Source: CAD feature listing. Evaluate the final solid. Frame: model axes, mm. Face numbers are marked on the shaded views. A direction names the side the tool comes from. Coordinates: 2 decimals unless noted, no trailing zeros. Loops run counter-clockwise (first coordinate to the right, second up) from the corner with the lowest first, then second, coordinate; pieces in that order, holes last.
Item 1: Pin query (flat end, axial travel): pin 1 Ø0.8 at (x, z) = (2.5, 16.5) entering from +Y; pin 2 Ø0.8 at (x, z) = (-3, 22) entering from -Y; pin 3 Ø2 at (y, z) = (2, 17) entering from -X; pin 4 Ø1.9 at (x, y) = (-6, 0) entering from -Z (3 decimals). Return the tip coordinate at first contact, or that it passes through.
Item 2: Reachability of the marked faces 5, 6, 7, 8 and 9 from +Z, -Z, +X, -X, +Y, -Y: full face, straight path, thin tool, end or side. Return the list, or none.
Item 3: Section query B-B, the plane z = 17. Return the cut outline in (x, y), then the cut area to 3 significant figures.
Item 4: Section query A-A, the plane x = 0. Return the cut outline in (y, z), then the cut area to 3 significant figures.
Item 5: Section query C-C, the plane y = 6. Return the cut outline in (x, z), then the cut area to 3 significant figures.
Item 6: Section query D-D, the plane x = -6.5. Return the cut outline in (y, z).
Item 7: Line query: probe 1 along Z at (x, y) = (2.5, -7); probe 2 along Y at (x, z) = (6, 0.65); probe 3 along Y at (x, z) = (4, 21.5). Output: solid intervals per line, ascending.
Item 8: Pull-direction query (Y, two-part tool) for the marked faces 1, 2, 3 and 4; classes: +Y half, -Y half, draft (parallel to the pull), parting line (faces both ways), or undercut.
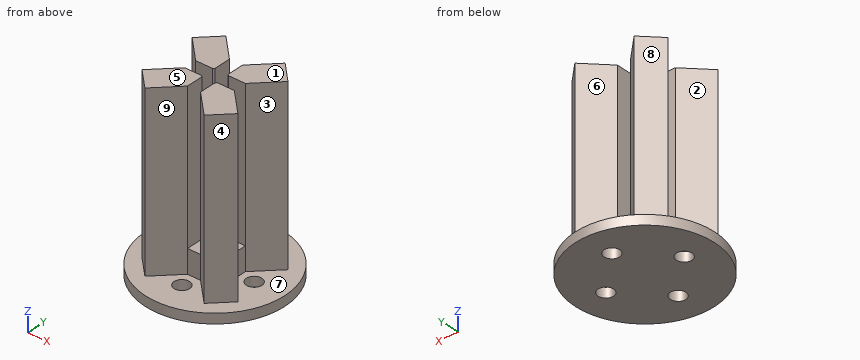
```python
from build123d import *

# Parameters (mm, degrees)
F0_R     = 10.66798
F1_DEPTH = 1.5
F2_R     = 1.19378
F3_DEPTH = 1.501
F4_W     = 7.606
F4_H     = 7.606
F5_DEPTH = 3.6
F6_W     = 2.803
F6_H     = 2.803
F7_DEPTH = 22.606
F9_DEPTH = 26.206
F10_SIZE = 0.2


with BuildPart() as f1:
    # F0 (on Top) → F1 (new body)
    with BuildSketch(Plane.XY):
        Circle(F0_R)
    extrude(amount=F1_DEPTH)

    # F2 (on face) → F3 (cut, through all)
    with BuildSketch(Plane.XY.offset(1.5)):
        with Locations((-6, 0)):
            Circle(F2_R)
        with Locations((0, 6)):
            Circle(F2_R)
        with Locations((6, 0)):
            Circle(F2_R)
        with Locations((0, -6)):
            Circle(F2_R)
    extrude(amount=-F3_DEPTH, mode=Mode.SUBTRACT)

    # F4 (on face) → F5 (join)
    with BuildSketch(Plane.XY.offset(1.5)):
        Rectangle(F4_W, F4_H)
    extrude(amount=F5_DEPTH)

    # F6 (on face) → F7 (join)
    with BuildSketch(Plane.XY.offset(5.1)):
        with Locations((-2.4015, 2.4015)):
            Rectangle(F6_W, F6_H)
        with Locations((-2.4015, -2.4015)):
            Rectangle(F6_W, F6_H)
        with Locations((2.4015, -2.4015)):
            Rectangle(F6_W, F6_H)
        with Locations((2.4015, 2.4015)):
            Rectangle(F6_W, F6_H)
    extrude(amount=F7_DEPTH)

    # F8 (on face) → F9 (join, through all)
    with BuildSketch(Plane.XY.offset(1.5)):
        Polygon((3.803, -3.803), (1, -3.803), (4.535534, -7.338534), (7.338534, -4.535534), (3.803, -1), align=None)
        Polygon((7.338534, 4.535534), (4.535534, 7.338534), (1, 3.803), (3.803, 3.803), (3.803, 1), align=None)
        Polygon((-4.535534, 7.338534), (-7.338534, 4.535534), (-3.803, 1), (-3.803, 3.803), (-1, 3.803), align=None)
        Polygon((-7.338534, -4.535534), (-4.535534, -7.338534), (-1, -3.803), (-3.803, -3.803), (-3.803, -1), align=None)
    extrude(amount=F9_DEPTH)

    # F10
    f10_edges = [f1.edges().sort_by_distance(p)[0] for p in [
        (-1, 1, 16.403),
        (1, 1, 16.403),
        (1, -1, 16.403),
        (-1, -1, 16.403),
    ]]
    chamfer(f10_edges, length=F10_SIZE)


solid = f1.part
```
Verdict:
1. pin 1: stops at y = 5.7
1. pin 2: stops at y = -6.2
1. pin 3: stops at x = -5.8
1. pin 4: passes through
2. face 5: +Z, +X, -X, +Y, -Y
2. face 6: +Z, +Y
2. face 7: +Z
2. face 8: +Z, -X, +Y
2. face 9: +Z, -Y
3. outline: (-7.34, -4.54) - (-4.54, -7.34) - (-1, -3.8) - (-1, -1.2) - (-1.2, -1) - (-3.8, -1) - close; (-7.34, 4.54) - (-3.8, 1) - (-1.2, 1) - (-1, 1.2) - (-1, 3.8) - (-4.54, 7.34) - close; (1, -3.8) - (4.54, -7.34) - (7.34, -4.54) - (3.8, -1) - (1.2, -1) - (1, -1.2) - close; (1, 1.2) - (1.2, 1) - (3.8, 1) - (7.34, 4.54) - (4.54, 7.34) - (1, 3.8) - close
3. area: 94.9 mm2
4. outline: (-10.67, 0) - (-7.19, 0) - (-7.19, 1.5) - (-10.67, 1.5) - close; (-4.81, 0) - (4.81, 0) - (4.81, 1.5) - (3.8, 1.5) - (3.8, 5.1) - (-3.8, 5.1) - (-3.8, 1.5) - (-4.81, 1.5) - close; (7.19, 0) - (10.67, 0) - (10.67, 1.5) - (7.19, 1.5) - close
4. area: 52.2 mm2
5. outline: (-8.82, 0) - (-1.19, 0) - (-1.19, 1.5) - (-3.2, 1.5) - (-3.2, 27.71) - (-5.87, 27.71) - (-5.87, 1.5) - (-8.82, 1.5) - close; (1.19, 0) - (8.82, 0) - (8.82, 1.5) - (5.87, 1.5) - (5.87, 27.71) - (3.2, 27.71) - (3.2, 1.5) - (1.19, 1.5) - close
5. area: 163 mm2
6. outline: (-8.46, 0) - (-1.08, 0) - (-1.08, 1.5) - (-3.7, 1.5) - (-3.7, 27.71) - (-5.37, 27.71) - (-5.37, 1.5) - (-8.46, 1.5) - close; (1.08, 0) - (8.46, 0) - (8.46, 1.5) - (5.37, 1.5) - (5.37, 27.71) - (3.7, 27.71) - (3.7, 1.5) - (1.08, 1.5) - close
7. probe 1: z = 0 to 1.5
7. probe 2: y = -8.82 to -1.19, 1.19 to 8.82
7. probe 3: y = -6.8 to -1.2, 1.2 to 6.8
8. face 1: draft
8. face 2: undercut
8. face 3: undercut
8. face 4: -Y half
